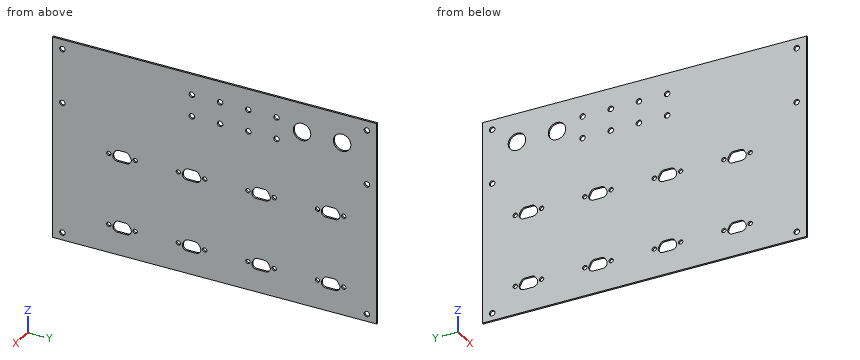
```python
from build123d import *

# Parameters (mm, degrees)
ESBO_O1_W                = 113.35
ESBO_O1_H                = 178.55
ESBO_O1_R                = 1.49999954
ESBO_O1_R_2              = 1.18
ESBO_O1_R_3              = 4.75
ESBO_O1_R_4              = 1.5
RESSALTO_EXTRUS_O2_DEPTH = 1
ESBO_O2_W                = 113.35
ESBO_O2_H                = 178.55
ESBO_O2_W_2              = 111.35
ESBO_O2_H_2              = 176.55
CORTE_EXTRUS_O1_DEPTH    = 586.381527556


with BuildPart() as part:
    # Esboço1 → Ressalto-extrusão2 (new body)
    with BuildSketch(Plane(origin=(0, 0, 0), x_dir=(0, 0, -1), z_dir=(1, 0, 0))):
        with Locations((-487.399286861, -126.719683222)):
            Rectangle(ESBO_O1_W, ESBO_O1_H)
        with Locations((-507.824286861, -209.584683222)):
            Circle(ESBO_O1_R, mode=Mode.SUBTRACT)
        with Locations((-537.796286861, -209.584683222)):
            Circle(ESBO_O1_R, mode=Mode.SUBTRACT)
        with Locations((-537.796286861, -43.722683222)):
            Circle(ESBO_O1_R, mode=Mode.SUBTRACT)
        with Locations((-507.824286861, -43.722683222)):
            Circle(ESBO_O1_R, mode=Mode.SUBTRACT)
        with Locations((-486.710286861, -56.312683222)):
            Circle(ESBO_O1_R_2, mode=Mode.SUBTRACT)
        with Locations((-486.710286861, -70.662683222)):
            Circle(ESBO_O1_R_2, mode=Mode.SUBTRACT)
        with Locations((-447.319286861, -70.662683222)):
            Circle(ESBO_O1_R_2, mode=Mode.SUBTRACT)
        with Locations((-447.319286861, -56.312683222)):
            Circle(ESBO_O1_R_2, mode=Mode.SUBTRACT)
        with Locations((-447.319286861, -94.184349889)):
            Circle(ESBO_O1_R_2, mode=Mode.SUBTRACT)
        with Locations((-447.319286861, -132.056016555)):
            Circle(ESBO_O1_R_2, mode=Mode.SUBTRACT)
        with Locations((-447.319286861, -108.534349889)):
            Circle(ESBO_O1_R_2, mode=Mode.SUBTRACT)
        with Locations((-447.319286861, -146.406016555)):
            Circle(ESBO_O1_R_2, mode=Mode.SUBTRACT)
        with Locations((-447.319286861, -184.277683222)):
            Circle(ESBO_O1_R_2, mode=Mode.SUBTRACT)
        with Locations((-447.319286861, -169.927683222)):
            Circle(ESBO_O1_R_2, mode=Mode.SUBTRACT)
        with Locations((-486.710286861, -184.277683222)):
            Circle(ESBO_O1_R_2, mode=Mode.SUBTRACT)
        with Locations((-486.710286861, -169.927683222)):
            Circle(ESBO_O1_R_2, mode=Mode.SUBTRACT)
        with Locations((-486.710286861, -146.406016555)):
            Circle(ESBO_O1_R_2, mode=Mode.SUBTRACT)
        with Locations((-486.710286861, -132.056016555)):
            Circle(ESBO_O1_R_2, mode=Mode.SUBTRACT)
        with Locations((-486.710286861, -94.184349889)):
            Circle(ESBO_O1_R_2, mode=Mode.SUBTRACT)
        with Locations((-486.710286861, -108.534349889)):
            Circle(ESBO_O1_R_2, mode=Mode.SUBTRACT)
        with Locations((-527.356886861, -79.028683222)):
            Circle(ESBO_O1_R_3, mode=Mode.SUBTRACT)
        with Locations((-527.356886861, -57.210083222)):
            Circle(ESBO_O1_R_3, mode=Mode.SUBTRACT)
        with Locations((-531.668289241, -139.043883661)):
            Circle(ESBO_O1_R_4, mode=Mode.SUBTRACT)
        with Locations((-531.668289241, -123.676879267)):
            Circle(ESBO_O1_R_4, mode=Mode.SUBTRACT)
        with Locations((-531.668289241, -108.309882502)):
            Circle(ESBO_O1_R_4, mode=Mode.SUBTRACT)
        with Locations((-531.668289241, -92.942885737)):
            Circle(ESBO_O1_R_4, mode=Mode.SUBTRACT)
        with Locations((-519.668289241, -92.942885737)):
            Circle(ESBO_O1_R_4, mode=Mode.SUBTRACT)
        with Locations((-519.668289241, -108.309882502)):
            Circle(ESBO_O1_R_4, mode=Mode.SUBTRACT)
        with Locations((-519.668289241, -123.676879267)):
            Circle(ESBO_O1_R_4, mode=Mode.SUBTRACT)
        with Locations((-519.668289241, -139.043883661)):
            Circle(ESBO_O1_R_4, mode=Mode.SUBTRACT)
        with Locations((-435.824286861, -209.584683222)):
            Circle(ESBO_O1_R_4, mode=Mode.SUBTRACT)
        with Locations((-435.824286861, -43.722683222)):
            Circle(ESBO_O1_R_4, mode=Mode.SUBTRACT)
        with BuildLine():
            Line((-489.835286861, -178.932542391), (-489.835286861, -175.272824053))
            ThreePointArc((-489.835286861, -175.272824053), (-489.499010625, -174.017824053), (-488.580286861, -173.09910029))
            Line((-488.580286861, -173.09910029), (-487.350286861, -172.388959458))
            ThreePointArc((-487.350286861, -172.388959458), (-484.840286861, -172.388959458), (-483.585286861, -174.562683222))
            Line((-483.585286861, -174.562683222), (-483.585286861, -179.642683222))
            ThreePointArc((-483.585286861, -179.642683222), (-484.840286861, -181.816406985), (-487.350286861, -181.816406985))
            Line((-487.350286861, -181.816406985), (-488.580286861, -181.106266154))
            ThreePointArc((-488.580286861, -181.106266154), (-489.499010625, -180.187542391), (-489.835286861, -178.932542391))
        make_face(mode=Mode.SUBTRACT)
        with BuildLine():
            Line((-487.350286861, -143.944740319), (-488.580286861, -143.234599488))
            ThreePointArc((-488.580286861, -143.234599488), (-489.499010625, -142.315875724), (-489.835286861, -141.060875724))
            Line((-489.835286861, -141.060875724), (-489.835286861, -137.401157386))
            ThreePointArc((-489.835286861, -137.401157386), (-489.499010625, -136.146157386), (-488.580286861, -135.227433623))
            Line((-488.580286861, -135.227433623), (-487.350286861, -134.517292792))
            ThreePointArc((-487.350286861, -134.517292792), (-484.840286861, -134.517292792), (-483.585286861, -136.691016555))
            Line((-483.585286861, -136.691016555), (-483.585286861, -141.771016555))
            ThreePointArc((-483.585286861, -141.771016555), (-484.840286861, -143.944740319), (-487.350286861, -143.944740319))
        make_face(mode=Mode.SUBTRACT)
        with BuildLine():
            Line((-488.580286861, -105.362932821), (-487.350286861, -106.073073652))
            ThreePointArc((-487.350286861, -106.073073652), (-484.840286861, -106.073073652), (-483.585286861, -103.899349889))
            Line((-483.585286861, -103.899349889), (-483.585286861, -98.819349889))
            ThreePointArc((-483.585286861, -98.819349889), (-484.840286861, -96.645626125), (-487.350286861, -96.645626125))
            Line((-487.350286861, -96.645626125), (-488.580286861, -97.355766956))
            ThreePointArc((-488.580286861, -97.355766956), (-489.499010625, -98.27449072), (-489.835286861, -99.52949072))
            Line((-489.835286861, -99.52949072), (-489.835286861, -103.189209058))
            ThreePointArc((-489.835286861, -103.189209058), (-489.499010625, -104.444209058), (-488.580286861, -105.362932821))
        make_face(mode=Mode.SUBTRACT)
        with BuildLine():
            Line((-489.835286861, -65.317542391), (-489.835286861, -61.657824053))
            ThreePointArc((-489.835286861, -61.657824053), (-489.499010625, -60.402824053), (-488.580286861, -59.48410029))
            Line((-488.580286861, -59.48410029), (-487.350286861, -58.773959458))
            ThreePointArc((-487.350286861, -58.773959458), (-484.840286861, -58.773959458), (-483.585286861, -60.947683222))
            Line((-483.585286861, -60.947683222), (-483.585286861, -66.027683222))
            ThreePointArc((-483.585286861, -66.027683222), (-484.840286861, -68.201406985), (-487.350286861, -68.201406985))
            Line((-487.350286861, -68.201406985), (-488.580286861, -67.491266154))
            ThreePointArc((-488.580286861, -67.491266154), (-489.499010625, -66.572542391), (-489.835286861, -65.317542391))
        make_face(mode=Mode.SUBTRACT)
        with BuildLine():
            Line((-447.959286861, -68.201406985), (-449.189286861, -67.491266154))
            ThreePointArc((-449.189286861, -67.491266154), (-450.108010625, -66.572542391), (-450.444286861, -65.317542391))
            Line((-450.444286861, -65.317542391), (-450.444286861, -61.657824053))
            ThreePointArc((-450.444286861, -61.657824053), (-450.108010625, -60.402824053), (-449.189286861, -59.48410029))
            Line((-449.189286861, -59.48410029), (-447.959286861, -58.773959458))
            ThreePointArc((-447.959286861, -58.773959458), (-445.449286861, -58.773959458), (-444.194286861, -60.947683222))
            Line((-444.194286861, -60.947683222), (-444.194286861, -66.027683222))
            ThreePointArc((-444.194286861, -66.027683222), (-445.449286861, -68.201406985), (-447.959286861, -68.201406985))
        make_face(mode=Mode.SUBTRACT)
        with BuildLine():
            Line((-450.444286861, -103.189209058), (-450.444286861, -99.52949072))
            ThreePointArc((-450.444286861, -99.52949072), (-450.108010625, -98.27449072), (-449.189286861, -97.355766956))
            Line((-449.189286861, -97.355766956), (-447.959286861, -96.645626125))
            ThreePointArc((-447.959286861, -96.645626125), (-445.449286861, -96.645626125), (-444.194286861, -98.819349889))
            Line((-444.194286861, -98.819349889), (-444.194286861, -103.899349889))
            ThreePointArc((-444.194286861, -103.899349889), (-445.449286861, -106.073073652), (-447.959286861, -106.073073652))
            Line((-447.959286861, -106.073073652), (-449.189286861, -105.362932821))
            ThreePointArc((-449.189286861, -105.362932821), (-450.108010625, -104.444209058), (-450.444286861, -103.189209058))
        make_face(mode=Mode.SUBTRACT)
        with BuildLine():
            Line((-449.189286861, -143.234599488), (-447.959286861, -143.944740319))
            ThreePointArc((-447.959286861, -143.944740319), (-445.449286861, -143.944740319), (-444.194286861, -141.771016555))
            Line((-444.194286861, -141.771016555), (-444.194286861, -136.691016555))
            ThreePointArc((-444.194286861, -136.691016555), (-445.449286861, -134.517292792), (-447.959286861, -134.517292792))
            Line((-447.959286861, -134.517292792), (-449.189286861, -135.227433623))
            ThreePointArc((-449.189286861, -135.227433623), (-450.108010625, -136.146157386), (-450.444286861, -137.401157386))
            Line((-450.444286861, -137.401157386), (-450.444286861, -141.060875724))
            ThreePointArc((-450.444286861, -141.060875724), (-450.108010625, -142.315875724), (-449.189286861, -143.234599488))
        make_face(mode=Mode.SUBTRACT)
        with BuildLine():
            Line((-450.444286861, -178.932542391), (-450.444286861, -175.272824053))
            ThreePointArc((-450.444286861, -175.272824053), (-450.108010625, -174.017824053), (-449.189286861, -173.09910029))
            Line((-449.189286861, -173.09910029), (-447.959286861, -172.388959458))
            ThreePointArc((-447.959286861, -172.388959458), (-445.449286861, -172.388959458), (-444.194286861, -174.562683222))
            Line((-444.194286861, -174.562683222), (-444.194286861, -179.642683222))
            ThreePointArc((-444.194286861, -179.642683222), (-445.449286861, -181.816406985), (-447.959286861, -181.816406985))
            Line((-447.959286861, -181.816406985), (-449.189286861, -181.106266154))
            ThreePointArc((-449.189286861, -181.106266154), (-450.108010625, -180.187542391), (-450.444286861, -178.932542391))
        make_face(mode=Mode.SUBTRACT)
    extrude(amount=RESSALTO_EXTRUS_O2_DEPTH)

    # Esboço2 → Corte-extrusão1 (cut, through all)
    with BuildSketch(Plane(origin=(1, 0, 0), x_dir=(0, 0, -1), z_dir=(1, 0, 0))):
        with Locations((-487.399286861, -126.719683222)):
            Rectangle(ESBO_O2_W, ESBO_O2_H)
        with Locations((-487.399286861, -126.719683222)):
            Rectangle(ESBO_O2_W_2, ESBO_O2_H_2, mode=Mode.SUBTRACT)
    extrude(amount=-CORTE_EXTRUS_O1_DEPTH, mode=Mode.SUBTRACT)


solid = part.part
```
Geometry check sheet. Reference: the model listing, model coordinates, mm. Coordinates: 2 decimals unless noted, no trailing zeros. Order: outer loops, then holes, each group sorted by start corner. A loop starts at its lowest first (then second) coordinate and runs counter-clockwise, first axis right, second up. Notation, with made-up numbers: (73, 16) - (105, 16) arc R17 cw to (105, 45) - close; hole circle Ø9 at (82, -6). An arc over 180 degrees is marked (long way). Answer as a JSON object with one key per item and string values. Group by question number.
Item 1: Sectioned sample at B-B, the plane x = 0.7. Give the number of separate pieces and of enclosed holes in the cut face, and give its area (3 significant figures).
Item 2: Sectioned sample at A-A, the plane z = 525.5. Record the cut outline in (x, y), and give its area (3 significant figures).
Item 3: Scan lines: probe 1 along Y at (x, z) = (0.85, 527.5); probe 2 along Z at (x, y) = (0.35, -97.5); probe 3 along Z at (x, y) = (0.6, -61.5). Record each from-to range of solid material in increasing order.
Item 4: Depth check by flat-ended pin: pin 1 Ø3 at (y, z) = (-83.5, 450) entering from -X. Enter the tip coordinate at first touch or a pass-through.
Resolved:
{
 "1": {"separate pieces": "1", "enclosed holes": "40", "area": "18,900 mm^2"},
 "2": {"outline": "(0, -214.99) - (1, -214.99) - (1, -83.4) - (0, -83.4) - close; (0, -74.66) - (1, -74.66) - (1, -61.58) - (0, -61.58) - close; (0, -52.84) - (1, -52.84) - (1, -38.44) - (0, -38.44) - close", "area": "159 mm^2"},
 "3": {"probe 1": "-214.99 to -83.78, -74.28 to -61.96, -52.46 to -38.44", "probe 2": "431.72 to 444.57, 449.41 to 483.96, 488.8 to 543.07", "probe 3": "431.72 to 444.19, 450.44 to 483.59, 489.83 to 525.32, 529.4 to 543.07"},
 "4": {"pin 1": "x = 0"}
}
